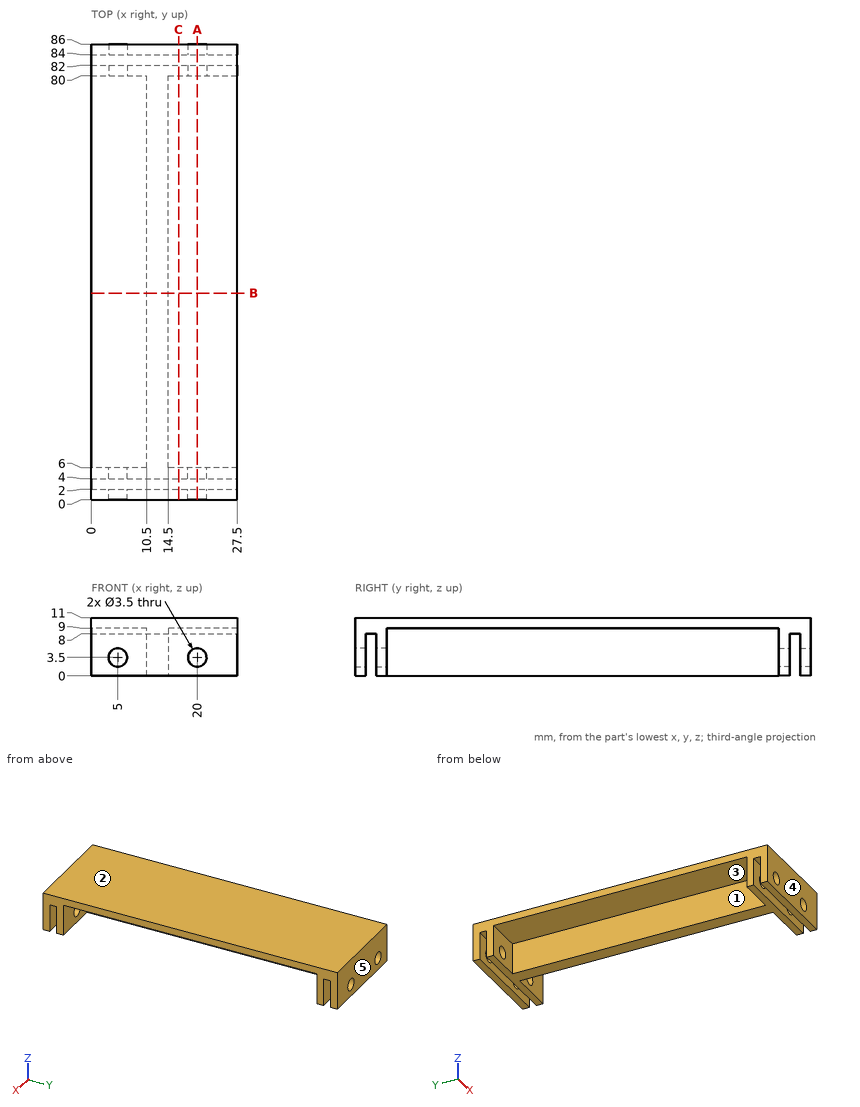
Can you work these out from the drawing? Everything is in mm from the part's minimum corner. A direction names the side the tool comes from. Round coordinates to 2 decimals unless told otherwise and drop trailing zeros. Loops run counter-clockwise (first coordinate to the right, second up) from the corner with the lowest first, then second, coordinate; pieces in that order, holes last. Notation, with made-up numbers: (84, 0) -> (135, 0) arc R9 cw to (135, 13) -> close; hole circle Ø5 at (44, 44.25). An arc over 180 degrees is marked (long way). Use CSV: the item, a comma, the result in double quotes.
(1) For the marked faces 1 and 2, which set-ups out of +Z, -Z, +X, -X, +Y, -Y let a thin tool reach every point of the face, with its end or its side?
Return value:
face 1,"-Z, -X"
face 2,"+Z, +X, -X, +Y, -Y"
(2) Suppose I cut it at B-B on y = 39. Write out the boundary of the cut face in (x, z).
Return value:
outline,"(0, 9) -> (10.5, 9) -> (10.5, 0) -> (14.5, 0) -> (14.5, 9) -> (27.5, 9) -> (27.5, 11) -> (0, 11) -> close"
(3) Suppose I cut it at A-A on x = 20. Give the number of separate pieces and of enclosed holes in the cut face, plus the area to 3 significant figures.
Return value:
separate pieces,"5"
enclosed holes,"0"
area,"220 mm²"
(4) If we mould it in two halves opening along Y, with no side actions, what happens to the marked faces 3, 4 and 5? For each: +Y half, -Y half, draft (parallel to the pull), parting line (faces both ways), or undercut.
Return value:
face 3,"undercut"
face 4,"-Y half"
face 5,"+Y half"
(5) Will these pins go through, and if not, where does the flat tip stop? pin 1 Ø1.5 at (x, y) = (23.5, 38.5) entering from -Z; pin 2 Ø2.5 at (x, z) = (23, 3.5) entering from -Y; pin 3 Ø3 at (x, z) = (5, 3.5) entering from -Y; pin 4 Ø4.5 at (y, z) = (45.5, 5) entering from -X.
Return value:
pin 1,"stops at z = 9"
pin 2,"stops at y = 0"
pin 3,"passes through"
pin 4,"stops at x = 10.5"
(6) If I drill on probe 1 along Y at (x, z) = (26.25, 1); probe 2 along X at (y, z) = (5.6, 3.5); probe 3 along Z at (x, y) = (5, 81.3), over which ranges is the centre line in solid material (lowest first)? Write a range as [from, to].
Return value:
probe 1,"y = [0, 2], [4, 6], [80, 82], [84, 86]"
probe 2,"x = [0, 3.25], [6.75, 18.25], [21.75, 27.5]"
probe 3,"z = [0, 1.75], [5.25, 11]"
(7) Suppose I cut it at C-C on x = 16.5. Write out the boundary of the cut face in (y, z), plus the area to 3 significant figures.
Return value:
outline,"(0, 0) -> (2, 0) -> (2, 8) -> (4, 8) -> (4, 0) -> (6, 0) -> (6, 9) -> (80, 9) -> (80, 0) -> (82, 0) -> (82, 8) -> (84, 8) -> (84, 0) -> (86, 0) -> (86, 11) -> (0, 11) -> close"
area,"248 mm²"
